Read the model definition and answer for the solid it produces. Units are mm, in the model's axes. Face numbers are marked on the shaded views. A direction names the side the tool comes from. Coordinates: 2 decimals unless noted, no trailing zeros. Write each loop counter-clockwise with the first axis right and the second up, starting at its lowest first coordinate (ties: lowest second). Pieces come first, ordered by that corner, then holes. Notation, with made-up numbers: (40.25, 74) -> (48.25, 74) arc R13 ccw to (48.25, 95) -> close; hole circle Ø5 at (75.5, -6). An arc over 180 degrees is marked (long way). One line per item, written item: value. Start each with the question number.
1. Consider line 1 along X through (y, z) = (31.5, -2.5); line 2 along Y through (x, z) = (15.5, -29.5); line 3 along Y through (x, z) = (3.5, 45). Determine where each line is inside the solid, lowest interval first.
2. Find section B-B, the plane z = -9.5. Write down the section's boundary in (x, y).
3. Given P1, Ø10, axis at x = 19.5, y = 86, coming from the -Z side; P2, Ø6.5, axis at x = 17.5, z = 18, coming from the +Y side; P3, Ø12, axis at y = 69, z = 12.5, coming from the -X side; P4, Ø16, axis at y = 19.5, z = 17.5, coming from the +X side, each flat-ended and moving along its own axis, determine where each tip first touches the part or whether it passes through.
4. For the marked faces 1, 2, 3 and 4, determine the directions among +Z, -Z, +X, -X, +Y, -Y from which every point of the face is accessible in a straight line to the end or side of a thin tool.
5. Find section A-A, the plane y = 47.5. Write down the section's boundary in (x, z), and give its area (3 significant figures).
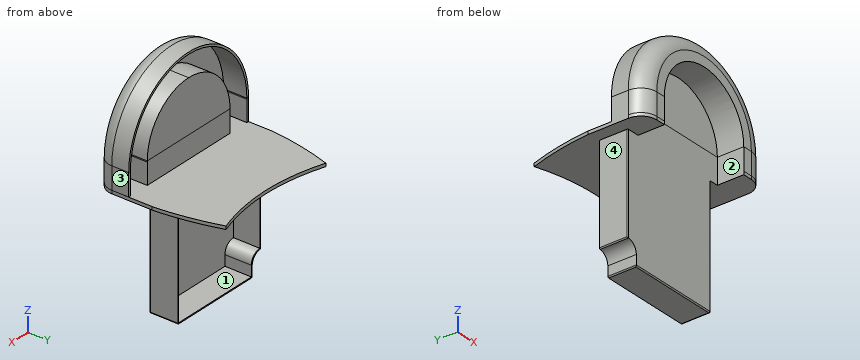
```python
from build123d import *

# Parameters (mm, degrees)
BOSS_EXTRUDE2_DEPTH      = 3
SKETCH14_W               = 98
SKETCH14_H               = 27.00264841
BOSS_EXTRUDE4_DEPTH      = 113
CUT_EXTRUDE11_DEPTH      = 25
BOSS_EXTRUDE5_DEPTH      = 21
REVOLVE1_ANGLE           = 180
CUT_EXTRUDE15_DEPTH      = 1
CUT_EXTRUDE15_DEPTH_BACK = 22
CUT_EXTRUDE14_DEPTH      = 24
CUT_REVOLVE2_ANGLE       = 180
CUT_EXTRUDE16_DEPTH      = 30
FILLET1_R                = 1


# Read off the part's stored shape, not the designer's step: Boss-Extrude5
with BuildPart() as part:
    # Sketch1 → Boss-Extrude2 (new body)
    with BuildSketch(Plane.XY):
        with BuildLine():
            Line((0, 0), (-55.99287927, 0.000657501))
            ThreePointArc((-55.99287927, 0.000657501), (-66.60214284, 4.395231334), (-70.996716676, 15.00467109))
            Line((-70.996716676, 15.00467109), (-70.996716676, 53.003088443))
            add(Edge.make_bspline(
                [(-59.092437552, 113.703738569), (-65.518680916, 93.709690833), (-69.486773958, 73.476140791), (-70.996716676, 53.003088443)],
                knots=[0.003076868, 0.003076868, 0.003076868, 0.003076868, 0.620649816, 0.620649816, 0.620649816, 0.620649816], degree=3))
            add(Edge.make_bspline(
                [(-59.092437552, 113.703738569), (-39.394984135, 107.237929235), (0.002749603, 100.771350363), (39.400586429, 107.237584193), (59.100918302, 113.704587579)],
                knots=[0.007529078, 0.007529078, 0.007529078, 0.007529078, 0.499976084, 0.992492475, 0.992492475, 0.992492475, 0.992492475], degree=3))
            add(Edge.make_bspline(
                [(59.100918302, 113.704587579), (65.524413648, 93.710040003), (69.490811091, 73.476198601), (71.000110633, 53.003063374)],
                knots=[0.003067815, 0.003067815, 0.003067815, 0.003067815, 0.620645861, 0.620645861, 0.620645861, 0.620645861], degree=3))
            Line((71.000110633, 53.003063374), (71.000110633, 15.004646021))
            ThreePointArc((71.000110633, 15.004646021), (66.605957202, 4.396221214), (55.998086385, 0.002067804))
            Line((55.998086385, 0.002067804), (0, 0))
        make_face()
    extrude(amount=BOSS_EXTRUDE2_DEPTH)

    # Sketch14 → Boss-Extrude4 (add)
    with BuildSketch(Plane(origin=(0, 0, 0), x_dir=(-1, 0, 0), z_dir=(0, 0, -1))):
        with Locations((10.005711619, 38.506146673)):
            Rectangle(SKETCH14_W, SKETCH14_H)
    extrude(amount=BOSS_EXTRUDE4_DEPTH)

    # Sketch17 → Cut-Extrude11 (cut)
    with BuildSketch(Plane(origin=(0, 52.007470878, 0), x_dir=(1, 0, 0), z_dir=(0, 1, 0))):
        with BuildLine():
            Line((-48.015549057, 109.013130471), (-48.015549057, 101.996525982))
            ThreePointArc((-48.015549057, 101.996525982), (-50.942812726, 94.929486331), (-58.009852377, 92.002222662))
            Line((-58.009852377, 92.002222662), (-58.009852377, 89.000786475))
            Line((-58.009852377, 89.000786475), (-58.009852377, 0))
            Line((-58.009852377, 0), (37.981980496, 0))
            Line((37.981980496, 0), (37.981980496, 111.996441685))
            Line((37.981980496, 111.996441685), (-48.015549057, 111.996441685))
            Line((-48.015549057, 111.996441685), (-48.015549057, 109.013130471))
        make_face()
    extrude(amount=-CUT_EXTRUDE11_DEPTH, mode=Mode.SUBTRACT)

    # Boss-Extrude5 outline → Boss-Extrude5 (add)
    with BuildSketch(Plane.XY.offset(3)):
        with BuildLine():
            Line((70.996140169, 31.00236483), (-70.996716676, 31.00236483))
            Line((-70.996716676, 31.00236483), (-70.996716676, 15.00467109))
            ThreePointArc((-70.996716676, 15.00467109), (-66.602205131, 4.395293626), (-55.99287927, 0.0006575))
            Line((-55.99287927, 0.0006575), (55.993738248, 0.002091992))
            ThreePointArc((55.993738248, 0.002091992), (66.60204984, 4.396315904), (70.996140169, 15.004682829))
            Line((70.996140169, 15.004682829), (70.996140169, 31.00236483))
        make_face()
    extrude(amount=BOSS_EXTRUDE5_DEPTH)

    # Sketch23 → Revolve1 (revolve)
    with BuildSketch(Plane.XY.offset(24)):
        with BuildLine():
            Line((-0.000288253, 31.00236483), (0, 0))
            Line((0, 0), (-55.996899325, 0.000681852))
            ThreePointArc((-55.996899325, 0.000681852), (-66.603382969, 4.39414471), (-70.996716676, 15.000681851))
            Line((-70.996716676, 15.000681851), (-70.996716676, 15.00467109))
            Line((-70.996716676, 15.00467109), (-70.996716676, 31.00236483))
            Line((-70.996716676, 31.00236483), (-0.000288253, 31.00236483))
        make_face()
    revolve(axis=Axis((-0.000288253, 31.00236483, 24), (-9.297785566939823e-06, 0.9999999999567756, 0)), revolution_arc=REVOLVE1_ANGLE)

    # Sketch24 → Cut-Extrude15 (cut, two sides: drawn at the far end of the back side and taken through both)
    with BuildSketch(Plane(origin=(0, 31.00236483, 0), x_dir=(1, 0, 0), z_dir=(0, 1, 0)).offset(-CUT_EXTRUDE15_DEPTH_BACK)):
        with BuildLine():
            Line((68.999389406, -3), (48.994713166, -3))
            Line((48.994713166, -3), (48.994713166, -22.995821368))
            ThreePointArc((48.994713166, -22.995821368), (49.002483122, -23.497884055), (49.005108381, -24))
            Line((49.005108381, -24), (69.006686122, -24))
            ThreePointArc((69.006686122, -24), (69.004864469, -23.497897411), (68.999389406, -22.995821368))
            Line((68.999389406, -22.995821368), (68.999389406, -3))
        make_face()
        with BuildLine():
            Line((-49.004079193, -24), (-69.003422409, -24))
            ThreePointArc((-69.003422409, -24), (0.001631857, -93.004353523), (69.006686122, -24))
            Line((69.006686122, -24), (49.005108381, -24))
            ThreePointArc((49.005108381, -24), (34.65421123, -58.654415118), (0.001631857, -73.009744406))
            ThreePointArc((0.001631857, -73.009744406), (-34.65239206, -58.655205184), (-49.004079193, -24))
        make_face()
        with BuildLine():
            Line((-48.993683978, -3), (-68.996125693, -3))
            Line((-68.996125693, -3), (-68.996125693, -22.995821368))
            ThreePointArc((-68.996125693, -22.995821368), (-69.001600755, -23.497897411), (-69.003422409, -24))
            Line((-69.003422409, -24), (-49.004079193, -24))
            ThreePointArc((-49.004079193, -24), (-49.001453934, -23.497884055), (-48.993683978, -22.995821368))
            Line((-48.993683978, -22.995821368), (-48.993683978, -3))
        make_face()
    extrude(amount=CUT_EXTRUDE15_DEPTH + CUT_EXTRUDE15_DEPTH_BACK, mode=Mode.SUBTRACT)

    # Sketch21 → Cut-Extrude14 (cut)
    with BuildSketch(Plane(origin=(0, 0, 0), x_dir=(-1, 0, 0), z_dir=(0, 0, -1))):
        Polygon((-46.994052442, 0.001735318), (-46.994052442, 25.004822468), (0, 25.004822468), (46.999021514, 25.004822468), (46.999021514, 0.000551889), (0, 0), align=None)
    extrude(amount=-CUT_EXTRUDE14_DEPTH, mode=Mode.SUBTRACT)

    # Sketch26 → Cut-Revolve2 (revolve, cut)
    with BuildSketch(Plane(origin=(0, 0, 24), x_dir=(-1, 0, 0), z_dir=(0, 0, -1))):
        Polygon((-46.994052442, 25.004822468), (0.002484536, 25.004822468), (0, -0.975536805), (-46.994052442, -0.975536805), (-46.994052442, 0.001735318), align=None)
    revolve(axis=Axis((0, -0.975536805, 24), (9.56313097373021e-05, -0.9999999954273263, 0)), revolution_arc=CUT_REVOLVE2_ANGLE, mode=Mode.SUBTRACT)

    # Sketch27 → Cut-Extrude16 (cut)
    with BuildSketch(Plane(origin=(0, 52.007470878, 0), x_dir=(1, 0, 0), z_dir=(0, 1, 0))):
        with BuildLine():
            Line((-49.010012163, 113), (-49.010012163, 102.994608886))
            ThreePointArc((-49.010012163, 102.994608886), (-66.073738487, 95.926582018), (-59.005711619, 112.990308342))
            Line((-59.005711619, 112.990308342), (-59.005711619, 113.493786648))
            Line((-59.005711619, 113.493786648), (-49.010012163, 113.493786648))
            Line((-49.010012163, 113.493786648), (-49.010012163, 113))
        make_face()
    extrude(amount=-CUT_EXTRUDE16_DEPTH, mode=Mode.SUBTRACT)

    # Fillet1
    fillet1_edges = [part.edges().sort_by_distance(p)[0] for p in [
        (-49.010012163, 38.506146673, -113),
        (-59.005711619, 25.004822468, -46.499454715),
        (-59.005711619, 38.506146673, -92.99890943),
        (38.994288381, 25.004822468, -56.5),
        (38.994288381, 38.506146673, -113),
        (-5.007861891, 25.004822468, -113),
    ]]
    fillet(fillet1_edges, radius=FILLET1_R)


solid = part.part
```
Answer block:
1. line 1: x = -59.01 to -58.01, 37.98 to 38.99
1. line 2: y = 25 to 27.01
1. line 3: y = 25 to 31
2. outline: (-59.01, 26) arc R1 ccw to (-58.01, 25) -> (37.99, 25) arc R1 ccw to (38.99, 26) -> (38.99, 52.01) -> (37.98, 52.01) -> (37.98, 27.01) -> (-58.01, 27.01) -> (-58.01, 52.01) -> (-59.01, 52.01) -> close
3. P1: stops at z = 0
3. P2: stops at y = 31
3. P3: passes through
3. P4: stops at x = 71
4. face 1: +Y
4. face 2: -Z, -Y
4. face 3: +Z, -Z, +X, +Y, -Y
4. face 4: -Z, -X, +Y, -Y
5. outline: (-71, 0) -> (-59.01, 0) -> (-59.01, -92.04) arc R1 ccw to (-58.1, -93.04) arc R10 cw to (-49.01, -102.99) -> (-49.01, -112) arc R1 ccw to (-48.01, -113) -> (37.99, -113) arc R1 ccw to (38.99, -112) -> (38.99, 0) -> (71, 0) -> (71, 3) -> (-71, 3) -> close; hole (-58.01, -92) arc R9.99 cw to (-48.02, -102) -> (-48.02, -112) -> (37.98, -112) -> (37.98, 0) -> (-58.01, 0) -> close
5. area: 749 mm2
